Geometry check sheet. Reference: the model listing, model coordinates, mm. A direction names the side the tool comes from. Coordinates: 2 decimals unless noted, no trailing zeros. Write each loop counter-clockwise with the first axis right and the second up, starting at its lowest first coordinate (ties: lowest second). Pieces come first, ordered by that corner, then holes. Notation, with made-up numbers: (48, 13.25) -> (87, 13.25) arc R22 ccw to (87, 23.25) -> close; hole circle Ø5 at (-29.75, -8.5). An arc over 180 degrees is marked (long way). Answer in a Markdown table with one row per item. Add a question column.
1. Cross-section at C-C on z = 15. Record the cut outline in (x, y).
2. Cross-section at B-B on y = -7. Record the cut outline in (x, z).
3. Set-up check for faces 1 (the flat face through (-8.85, 11, -23)), 2 (the cylindrical face through (1.68, 21.29, -4.66)), 3 (the cylindrical face through (1.05, 22.02, -7.46)): record each of +Z, -Z, +X, -X, +Y, -Y from which the full face is reachable in a straight line by a thin tool's end or side.
4. Cross-section at A-A on z = 24. Record the cut outline in (x, y), and give its area (3 significant figures).
5. Scan lines: L1, parallel to X at y = 10, z = -24; L2, parallel to X at y = 24.05, z = -10; L3, parallel to Z at x = -3.25, y = -13.5. Record each from-to range of solid material in increasing order. Write a range as from..to.
6. Depth check by flat-ended pin: P1, Ø1, axis at y = 12.5, z = -24, coming from the +X side; P2, Ø2, axis at x = 6, z = 1.5, coming from the +Y side; P3, Ø2, axis at y = 11, z = -23.5, coming from the -X side. Enter the tip coordinate at first touch or a pass-through.
7. Mould release check, pull along Z, two halves, no side actions. Record for faces 4 (the flat face through (-3.9, 11, 26)), 5 (the cylindrical face through (8.4, 10.53, 26.57)), 6 (the cylindrical face through (4.93, 10.57, 22.1)): pulls with the +Z half, pulls with the -Z half, needs draft (parallel to the pull), parting line crosses it, or undercut.
8. Cross-section at D-D on z = -29.5. Record the cut outline in (x, y).
```python
from build123d import *
from OCP.BRepFilletAPI import BRepFilletAPI_MakeChamfer

# Parameters (mm, degrees)
SKETCH2_W                 = 19.5
SKETCH2_H                 = 40.5
BOSS_EXTRUDE1_DEPTH       = 17.8
CHAMFER1_SIZE             = 2.5
CHAMFER1_SIZE2            = 0.909925586
FILLET1_R                 = 1.5
BOSS_EXTRUDE2_START       = -6
SKETCH3_W                 = 17.7
SKETCH3_H                 = 54
BOSS_EXTRUDE2_DEPTH       = 2.5
FILLET2_R                 = 1.5
BOSS_EXTRUDE3_DEPTH       = 0.65
BOSS_EXTRUDE4_DEPTH       = 1.9
SKETCH6_R                 = 6.4
BOSS_EXTRUDE5_DEPTH       = 1.2
SKETCH7_R                 = 5.6
BOSS_EXTRUDE6_DEPTH       = 0.8
SKETCH8_R                 = 2.75
BOSS_EXTRUDE7_DEPTH       = 4
SKETCH9_R                 = 3
BOSS_EXTRUDE8_DEPTH       = 3.4
CHAMFER2_SIZE             = 0.3
CHAMFER3_SIZE             = 0.5
CUT_EXTRUDE1_REACH        = 43.234
MIRROR3_COPY_1_REACH      = 43.234
SKETCH12_W                = 6.8
SKETCH12_H                = 4
BOSS_EXTRUDE9_DEPTH       = 0.8
SKETCH13_W                = 6.4
SKETCH13_H                = 3.6
BOSS_EXTRUDE10_DEPTH      = 4.2
BOSS_EXTRUDE10_TAPER      = 3
BOSS_EXTRUDE11_DEPTH      = 10
M3X0_5_TAPPED_HOLE1_D     = 2.5
M3X0_5_TAPPED_HOLE1_DEPTH = 6
M3X0_5_TAPPED_HOLE1_TIP   = 0.751075774


with BuildPart() as part:
    # Sketch2 → Boss-Extrude1 (new, symmetric)
    with BuildSketch(Plane(origin=(0, 0, 0), x_dir=(1, 0, 0), z_dir=(0, 1, 0))):
        Rectangle(SKETCH2_W, SKETCH2_H)
    extrude(amount=BOSS_EXTRUDE1_DEPTH, both=True)

    # Chamfer1: one chamfer whose edges measure the first distance from different faces: ONE call of the kernel's chamfer builder (chamfer() names one face for all edges)
    chamfer1_edges_1 = [part.edges().sort_by_distance(p)[0] for p in [
        (0, -17.8, -20.25),
    ]]
    chamfer1_side_1 = [part.faces().sort_by_distance(p)[0] for p in [
        (0, 0, -20.25),
    ]]
    chamfer1_edges_2 = [part.edges().sort_by_distance(p)[0] for p in [
        (9.75, -17.8, 0),
    ]]
    chamfer1_side_2 = [part.faces().sort_by_distance(p)[0] for p in [
        (9.75, 0, 0),
    ]]
    chamfer1_edges_3 = [part.edges().sort_by_distance(p)[0] for p in [
        (0, -17.8, 20.25),
    ]]
    chamfer1_side_3 = [part.faces().sort_by_distance(p)[0] for p in [
        (0, 0, 20.25),
    ]]
    chamfer1_edges_4 = [part.edges().sort_by_distance(p)[0] for p in [
        (-9.75, -17.8, 0),
    ]]
    chamfer1_side_4 = [part.faces().sort_by_distance(p)[0] for p in [
        (-9.75, 0, 0),
    ]]
    chamfer1 = BRepFilletAPI_MakeChamfer(part.part.solid().wrapped)
    for e in chamfer1_edges_1:
        chamfer1.Add(CHAMFER1_SIZE, CHAMFER1_SIZE2, e.wrapped, chamfer1_side_1[0].wrapped)  # the first distance lies on this face
    for e in chamfer1_edges_2:
        chamfer1.Add(CHAMFER1_SIZE, CHAMFER1_SIZE2, e.wrapped, chamfer1_side_2[0].wrapped)  # the first distance lies on this face
    for e in chamfer1_edges_3:
        chamfer1.Add(CHAMFER1_SIZE, CHAMFER1_SIZE2, e.wrapped, chamfer1_side_3[0].wrapped)  # the first distance lies on this face
    for e in chamfer1_edges_4:
        chamfer1.Add(CHAMFER1_SIZE, CHAMFER1_SIZE2, e.wrapped, chamfer1_side_4[0].wrapped)  # the first distance lies on this face
    add(Compound.cast(chamfer1.Shape()), mode=Mode.REPLACE)

    # Fillet1
    # the kernel refuses this fillet: 1.5 mm, written as the material it takes off along each edge
    with BuildSketch(Plane(origin=(-10.829006934, -12.335452813, -21.329006934), x_dir=(0.9461886483394649, 0.3040991697893321, -0.11068304606838018), z_dir=(0.3236155771181854, -0.8891264907159878, 0.32361557711818534)), Plane(origin=(-10.829006934, -12.335452813, 21.329006934), x_dir=(-0.1106830460683806, 0.30409916978933194, -0.946188648339465), z_dir=(0.32361557711818534, -0.8891264907159879, -0.3236155771181854))) as fillet1_piece_1:
        with BuildLine():
            CenterArc((FILLET1_R * 0.889126490716, FILLET1_R), FILLET1_R, 186.717713464, 83.282286536)
            Line((-FILLET1_R * 0.104008041637, FILLET1_R * 0.883022221559), (0, 0))
            Line((0, 0), (FILLET1_R * 0.889126490716, 0))
        make_face()
    extrude(amount=9.480197094, mode=Mode.SUBTRACT)
    with BuildSketch(Plane(origin=(10.829006934, -12.335452813, -21.329006934), x_dir=(-0.946188648339465, 0.30409916978933194, -0.1106830460683806), z_dir=(-0.3236155771181854, -0.8891264907159879, 0.3236155771181854)), Plane(origin=(10.829006934, -12.335452813, 21.329006934), x_dir=(0.11068304606838136, 0.3040991697893317, -0.9461886483394651), z_dir=(-0.3236155771181854, -0.8891264907159879, -0.3236155771181854))) as fillet1_piece_2:
        with BuildLine():
            CenterArc((FILLET1_R * 0.889126490716, -FILLET1_R), FILLET1_R, 90, 83.282286536)
            Line((-FILLET1_R * 0.104008041637, -FILLET1_R * 0.883022221559), (0, 0))
            Line((0, 0), (FILLET1_R * 0.889126490716, 0))
        make_face()
    extrude(amount=9.480197094, mode=Mode.SUBTRACT)
    with BuildSketch(Plane(origin=(-9.75, -19.05, -20.25), x_dir=(1, 0, 0), z_dir=(0, 1, 0)), Plane(origin=(9.75, 21.55, -20.25), x_dir=(-1, 0, 0), z_dir=(0, -1, 0)), Plane(origin=(9.75, 21.55, 20.25), x_dir=(0, 0, -1), z_dir=(0, -1, 0)), Plane(origin=(-9.75, -19.05, 20.25), x_dir=(0, 0, -1), z_dir=(0, 1, 0))) as fillet1_piece_3:
        with BuildLine():
            CenterArc((FILLET1_R, -FILLET1_R), FILLET1_R, 90, 90)
            Line((0, -FILLET1_R), (0, 0))
            Line((0, 0), (FILLET1_R, 0))
        make_face()
    extrude(amount=40.6, mode=Mode.SUBTRACT)

    # Sketch3 → Boss-Extrude2 (add)
    with BuildSketch(Plane(origin=(0, 17.8, 0), x_dir=(1, 0, 0), z_dir=(0, 1, 0)).offset(BOSS_EXTRUDE2_START)):
        Rectangle(SKETCH3_W, SKETCH3_H)
    extrude(amount=-BOSS_EXTRUDE2_DEPTH)

    # Fillet2
    fillet2_edges = [part.edges().sort_by_distance(p)[0] for p in [
        (-8.85, 10.55, 27),
        (8.85, 10.55, -27),
        (-8.85, 10.55, -27),
        (8.85, 10.55, 27),
    ]]
    fillet(fillet2_edges, radius=FILLET2_R)

    # Sketch4 → Boss-Extrude3 (add, symmetric)
    with BuildSketch(Plane(origin=(0, 0, 0), x_dir=(0, 0, -1), z_dir=(1, 0, 0))):
        Polygon((-20.25, 11.8), (-27, 11.8), (-27, 12), (-20.25, 13.1), align=None)
    boss_extrude3 = extrude(amount=BOSS_EXTRUDE3_DEPTH, both=True)

    # Mirror1: Boss-Extrude3 across plane
    add(boss_extrude3.mirror(Plane.XY))

    # Sketch5 → Boss-Extrude4 (add)
    with BuildSketch(Plane(origin=(0, 17.8, 0), x_dir=(1, 0, 0), z_dir=(0, 1, 0))):
        with BuildLine():
            Line((-8.9, 6.01848019), (-8.9, -14.25))
            Line((-8.9, -14.25), (-4.5, -14.25))
            ThreePointArc((-4.5, -14.25), (0, -16.55), (4.5, -14.25))
            Line((4.5, -14.25), (8.9, -14.25))
            Line((8.9, -14.25), (8.9, 6.01848019))
            ThreePointArc((8.9, 6.01848019), (0, 19.75), (-8.9, 6.01848019))
        make_face()
    extrude(amount=BOSS_EXTRUDE4_DEPTH)

    # Sketch6 → Boss-Extrude5 (add)
    with BuildSketch(Plane(origin=(0, 19.7, 0), x_dir=(1, 0, 0), z_dir=(0, 1, 0))):
        with Locations(Location((0, 10, 0), (0, 0, 270))):
            Circle(SKETCH6_R)
    extrude(amount=BOSS_EXTRUDE5_DEPTH)

    # Sketch7 → Boss-Extrude6 (add)
    with BuildSketch(Plane(origin=(0, 20.9, 0), x_dir=(1, 0, 0), z_dir=(0, 1, 0))):
        with Locations(Location((0, 10, 0), (0, 0, 270))):
            Circle(SKETCH7_R)
    extrude(amount=BOSS_EXTRUDE6_DEPTH)

    # Sketch8 → Boss-Extrude7 (add)
    with BuildSketch(Plane(origin=(0, 21.7, 0), x_dir=(1, 0, 0), z_dir=(0, 1, 0))):
        with Locations(Location((0, 10, 0), (0, 0, 270))):
            Circle(SKETCH8_R)
    extrude(amount=BOSS_EXTRUDE7_DEPTH)

    # Sketch9 → Boss-Extrude8 (add)
    with BuildSketch(Plane(origin=(0, 25.7, 0), x_dir=(1, 0, 0), z_dir=(0, 1, 0))):
        with Locations(Location((0, 10, 0), (0, 0, 270))):
            Circle(SKETCH9_R)
    extrude(amount=-BOSS_EXTRUDE8_DEPTH)

    # Chamfer2
    # the kernel refuses this chamfer: 0.3 mm, written as the material it takes off along each edge
    with BuildSketch(Plane(origin=(0, 22.3, -10), x_dir=(0, 0, 1), z_dir=(-1, 0, 0))) as chamfer2_piece_1_section:
        Polygon((3 - CHAMFER2_SIZE, 0), (3, CHAMFER2_SIZE), (3, 0), align=None)
    chamfer2_piece_1 = revolve(axis=Axis((0, 22.3, -10), (0, 1, 0)), mode=Mode.PRIVATE)
    chamfer2_piece_1 = chamfer2_piece_1 - Plane(origin=(0, 22.47249354, -10), x_dir=(0, 0, 1), z_dir=(0, -1, 0)) * Cylinder(2.75, 12, mode=Mode.PRIVATE)
    add(chamfer2_piece_1, mode=Mode.SUBTRACT)

    # Chamfer3
    chamfer3_edges = [part.edges().sort_by_distance(p)[0] for p in [
        (0, 25.7, -13),
    ]]
    chamfer(chamfer3_edges, length=CHAMFER3_SIZE)

    # Sketch11 → Cut-Extrude1 (cut, up to next)
    with BuildSketch(Plane(origin=(0, 11.8, 0), x_dir=(1, 0, 0), z_dir=(0, 1, 0)), mode=Mode.PRIVATE) as cut_extrude1_sk1:
        with BuildLine():
            Line((6.1, -27), (3.9, -27))
            Line((3.9, -27), (3.9, -25.549193338))
            ThreePointArc((3.9, -25.549193338), (5, -22.1), (6.1, -25.549193338))
            Line((6.1, -25.549193338), (6.1, -27))
        make_face()
    cut_extrude1_tool1 = extrude(cut_extrude1_sk1.sketch, amount=-CUT_EXTRUDE1_REACH, mode=Mode.PRIVATE) & part.part
    cut_extrude1 = cut_extrude1_tool1.solids().sort_by_distance((5, 11.8, 24.454928))[0]
    add(cut_extrude1, mode=Mode.SUBTRACT)

    # Mirror2: Cut-Extrude1 across plane
    add(cut_extrude1.mirror(Plane(origin=(0, 0, 0), x_dir=(0, 0, 1), z_dir=(1, 0, 0))), mode=Mode.SUBTRACT)

    # Mirror3: Cut-Extrude1 across plane
    add(cut_extrude1.mirror(Plane.XY), mode=Mode.SUBTRACT)

    # Mirror3 copy 1 sketch → Mirror3 copy 1 (cut, up to next)
    with BuildSketch(Plane(origin=(0, 11.8, 0), x_dir=(-1, 0, 0), z_dir=(0, 1, 0)), mode=Mode.PRIVATE) as mirror3_copy_1_sk1:
        with BuildLine():
            Line((6.1, -27), (3.9, -27))
            Line((3.9, -27), (3.9, -25.549193338))
            ThreePointArc((3.9, -25.549193338), (5, -22.1), (6.1, -25.549193338))
            Line((6.1, -25.549193338), (6.1, -27))
        make_face()
    mirror3_copy_1_tool1 = extrude(mirror3_copy_1_sk1.sketch, amount=-MIRROR3_COPY_1_REACH, mode=Mode.PRIVATE) & part.part
    add(mirror3_copy_1_tool1.solids().sort_by_distance((-5, 11.8, -24.454928))[0], mode=Mode.SUBTRACT)

    # Sketch12 → Boss-Extrude9 (add)
    with BuildSketch(Plane.XY.offset(-20.25)):
        with Locations((0, -12.5)):
            Rectangle(SKETCH12_W, SKETCH12_H)
    extrude(amount=-BOSS_EXTRUDE9_DEPTH)

    # Sketch13 → Boss-Extrude10 (add)
    with BuildSketch(Plane(origin=(0, 0, -21.05), x_dir=(-1, 0, 0), z_dir=(0, 0, -1))):
        with Locations((0, -12.5)):
            Rectangle(SKETCH13_W, SKETCH13_H)
    extrude(amount=BOSS_EXTRUDE10_DEPTH, taper=BOSS_EXTRUDE10_TAPER)

    # Sketch14 → Boss-Extrude11 (add)
    with BuildSketch(Plane(origin=(0, 0, -25.25), x_dir=(-1, 0, 0), z_dir=(0, 0, -1))):
        with BuildLine():
            ThreePointArc((0.75, -12.778388218), (2.3, -12.5), (0.75, -12.221611782))
            ThreePointArc((0.75, -12.221611782), (0, -11.7), (-0.75, -12.221611782))
            ThreePointArc((-0.75, -12.221611782), (-2.3, -12.5), (-0.75, -12.778388218))
            ThreePointArc((-0.75, -12.778388218), (0, -13.3), (0.75, -12.778388218))
        make_face()
    extrude(amount=BOSS_EXTRUDE11_DEPTH)

    # M3x0.5 Tapped Hole1
    with Locations(Plane(origin=(0, 25.7, 0), x_dir=(1, 0, 0), z_dir=(0, 1, 0))):
        with Locations((0, 10)):
            Hole(M3X0_5_TAPPED_HOLE1_D / 2, depth=M3X0_5_TAPPED_HOLE1_DEPTH)
            with Locations((0, 0, -(M3X0_5_TAPPED_HOLE1_DEPTH + M3X0_5_TAPPED_HOLE1_TIP / 2))):  # 118° drill point
                Cone(0, M3X0_5_TAPPED_HOLE1_D / 2, M3X0_5_TAPPED_HOLE1_TIP, mode=Mode.SUBTRACT)


solid = part.part
```
Results found:
| question | item | result |
|---|---|---|
| 1 | outline | (-9.75, -15.3) -> (-8.84, -17.8) -> (8.84, -17.8) -> (9.75, -15.3) -> (9.75, 17.8) -> (3.85, 17.8) -> (3.85, 19.7) -> (-3.85, 19.7) -> (-3.85, 17.8) -> (-9.75, 17.8) -> close |
| 2 | outline | (-9.75, -18.75) arc R1.5 ccw to (-8.25, -20.25) -> (8.25, -20.25) arc R1.5 ccw to (9.75, -18.75) -> (9.75, 18.75) arc R1.5 ccw to (8.25, 20.25) -> (-8.25, 20.25) arc R1.5 ccw to (-9.75, 18.75) -> close |
| 3 | face 1 | -Z, -X, +Y, -Y |
| 3 | face 2 | +Y |
| 3 | face 3 | none |
| 4 | outline | (-8.85, 9.3) -> (-6.9, 9.3) -> (-6.9, 11.8) -> (-8.85, 11.8) -> close; (-3.1, 9.3) -> (3.1, 9.3) -> (3.1, 11.8) -> (0.65, 11.8) -> (0.65, 12.49) -> (-0.65, 12.49) -> (-0.65, 11.8) -> (-3.1, 11.8) -> close; (6.9, 9.3) -> (8.85, 9.3) -> (8.85, 11.8) -> (6.9, 11.8) -> close |
| 4 | area | 26.1 mm^2 |
| 5 | L1 | x = -8.85..-6.9, -3.1..3.1, 6.9..8.85 |
| 5 | L2 | x = -3..-1.25, 1.25..3 |
| 5 | L3 | z = -21.05..20.25 |
| 6 | P1 | stops at x = 0.65 |
| 6 | P2 | stops at y = 19.7 |
| 6 | P3 | stops at x = -8.85 |
| 7 | face 4 | needs draft |
| 7 | face 5 | pulls with the +Z half |
| 7 | face 6 | undercut |
| 8 | outline | (-0.75, -12.78) arc R0.8 ccw to (0.75, -12.78) arc R0.8 ccw (long way) to (0.75, -12.22) arc R0.8 ccw to (-0.75, -12.22) arc R0.8 ccw (long way) to start |
